```python
from build123d import *

# Parameters (mm, degrees)
SKETCH1_W     = 1.5
SKETCH1_H     = 50
FILLET1_R     = 0.5
CHAMFER1_SIZE = 0.5


with BuildPart() as part:
    # Sketch1 → Revolve1 (revolve)
    with BuildSketch(Plane.YZ):
        with Locations((0.75, 25)):
            Rectangle(SKETCH1_W, SKETCH1_H)
        Polygon((1.5, 0), (0, 0), (0, -2), (9, -2), (9, 0), align=None)
    revolve(axis=Axis((0, 0, -11.370061245), (0, 0, 1)))

    # Fillet1
    fillet1_edges = [part.edges().sort_by_distance(p)[0] for p in [
        (0, -1.5, 50),
    ]]
    fillet(fillet1_edges, radius=FILLET1_R)

    # Chamfer1
    chamfer1_edges = [part.edges().sort_by_distance(p)[0] for p in [
        (0, -9, 0),
    ]]
    chamfer(chamfer1_edges, length=CHAMFER1_SIZE)


solid = part.part
```
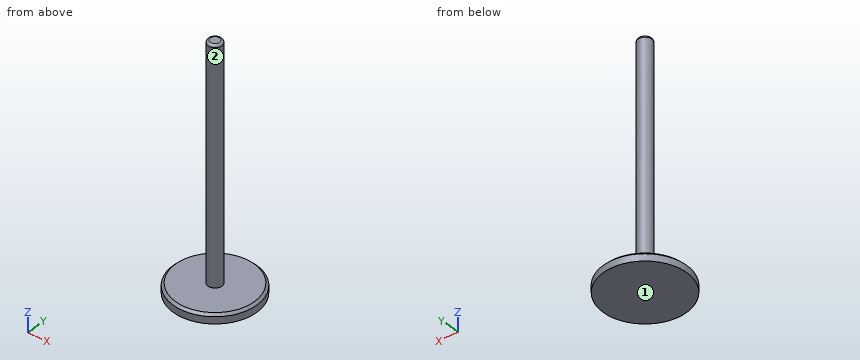
Here's how the part is built. I have some questions about the finished solid (model axes, mm). Face numbers are marked on the shaded views. A direction names the side the tool comes from. Coordinates: 2 decimals unless noted, no trailing zeros. Loops run counter-clockwise (first coordinate to the right, second up) from the corner with the lowest first, then second, coordinate; pieces in that order, holes last. Notation, with made-up numbers: M 85.5,0 L 140.5,0 A19 cw 140.5,30 Z; hole C 71,40.5 d6. An arc over 180 degrees is marked long. One line per item, written item: value.
1. Will these pins go through, and if not, where does the flat tip stop? pin 1 Ø2 at (x, z) = (1, 8) entering from -Y; pin 2 Ø10 at (x, z) = (-2.5, 41) entering from +Y; pin 3 Ø2 at (y, z) = (4, 27) entering from -X.
Geometry says:
pin 1: stops at y = -1.5
pin 2: stops at y = 1.5
pin 3: passes through
2. On a 3-axis mill with a long thin cutter (end or side, diameter ignored), from which of +Z, -Z, +X, -X, +Y, -Y can I reach the whole of each face in a straight line? I mean the marked faces 1 and 2. Say none if no direction works.
Geometry says:
face 1: -Z, +X, -X, +Y, -Y
face 2: +Z
3. Imagine slicing it at C-C (z = 18.5). List the corners of the cut face in (x, y) for me, and give its area (3 significant figures).
Geometry says:
outline: C 0,0 d3
area: 7.07 mm2
4. Please list where these lines run through material, in increasing order: probe 1 along Z at (x, y) = (-7.25, 2); probe 2 along Y at (x, z) = (1, 8); probe 3 along Y at (x, z) = (0.75, 41.5).
Geometry says:
probe 1: z = -2 to 0
probe 2: y = -1.12 to 1.12
probe 3: y = -1.3 to 1.3
5. Imagine slicing it at A-A (y = 0). List the corners of the cut face in (x, z) for me, and give its area (3 significant figures).
Geometry says:
outline: M -9,-2 L 9,-2 L 9,-0.5 L 8.5,0 L 1.5,0 L 1.5,49.5 A0.5 ccw 1,50 L -1,50 A0.5 ccw -1.5,49.5 L -1.5,0 L -8.5,0 L -9,-0.5 Z
area: 186 mm2
